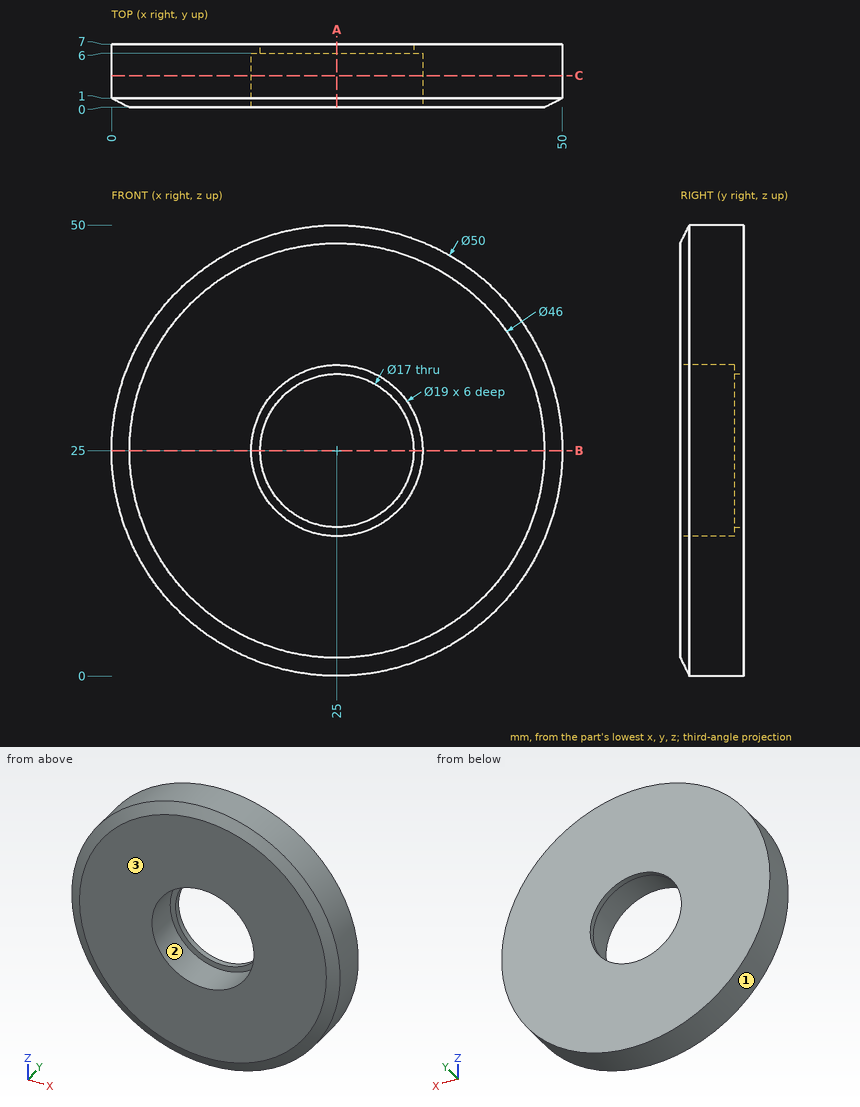
Can you work these out from the drawing? Everything is in mm from the part's minimum corner. Give positions to 0.01 mm unless a question says otherwise; leave off trailing zeros. Order: outer loops, then holes, each group sorted by start corner. A loop starts at its lowest first (then second) coordinate and runs counter-clockwise, first axis right, second up.
Item 1: If we section it at A-A, the plane x = 25: Write out the boundary of the cut face in (y, z).
Item 2: I'm going to push flat-ended pins straight in: pin 1 (5.5 mm diameter, centred on x = 29.5, z = 21.5, fed in from -Y); pin 2 (1.5 mm diameter, centred on x = 11, y = 4.5, fed in from +Z); pin 3 (3 mm diameter, centred on y = 2.5, z = 5.5, fed in from +X); pin 4 (1.5 mm diameter, centred on x = 38.5, y = 2, fed in from -Z). Where does each tip first touch, or does it pass through?
Item 3: If we section it at C-C, the plane y = 3.5: Write out the boundary of the cut face in (x, z).
Item 4: I need wall thicknesses on line 1 (Z direction, x = 25, y = 6.4); line 2 (Z direction, x = 25, y = 2.65); line 3 (X direction, y = 6.25, z = 24.5) (3 decimals). Which ranges of each line are inside material? Lowest first, please.
Item 5: If we mould it in two halves opening along X, with no side actions, what happens to the marked faces 1, 2 and 3? For each: pulls with the +X half, pulls with the -X half, needs draft (parallel to the pull), parting line crosses it, or undercut.
Item 6: If we section it at B-B, the plane z = 25: Write out the boundary of the cut face in (x, y).
Values:
1. outline: (0, 2) - (1, 0) - (7, 0) - (7, 16.5) - (6, 16.5) - (6, 15.5) - (0, 15.5) - close; (0, 34.5) - (6, 34.5) - (6, 33.5) - (7, 33.5) - (7, 50) - (1, 50) - (0, 48) - close
2. pin 1: passes through
2. pin 2: stops at z = 46.2
2. pin 3: stops at x = 42.35
2. pin 4: stops at z = 3.5
3. outline: circle Ø50 at (25, 25); hole circle Ø19 at (25, 25)
4. line 1: z = 0 to 16.5, 33.5 to 50
4. line 2: z = 0 to 15.5, 34.5 to 50
4. line 3: x = 0.005 to 16.515, 33.485 to 49.995
5. face 1: parting line crosses it
5. face 2: undercut
5. face 3: needs draft
6. outline: (0, 1) - (2, 0) - (15.5, 0) - (15.5, 6) - (16.5, 6) - (16.5, 7) - (0, 7) - close; (33.5, 6) - (34.5, 6) - (34.5, 0) - (48, 0) - (50, 1) - (50, 7) - (33.5, 7) - close
